Here's how the part is built. I have some questions about the finished solid (model axes, mm). Face numbers are marked on the shaded views. A direction names the side the tool comes from. Round coordinates to 2 decimals unless told otherwise and drop trailing zeros. Loops run counter-clockwise (first coordinate to the right, second up) from the corner with the lowest first, then second, coordinate; pieces in that order, holes last. Notation, with made-up numbers: (14, -33.5) - (66, -33.5) arc R22 ccw to (66, -9.5) - close; hole circle Ø2 at (78, 24.25). An arc over 180 degrees is marked (long way). Answer as a JSON object with one key per item and string values. Group by question number.
1) If I drill on line 1 along Z through (x, y) = (8.5, 1.05); line 2 along X through (y, z) = (21.5, -12.5) (3 decimals); line 3 along X through (y, z) = (17, -12) (3 decimals), over which ranges is the centre line in solid material (lowest first)? Write a range as [from, to].
2) Which directions (+Z, -Z, +X, -X, +Y, -Y) give clear straight access to the entire face, cutting with the end or side of a thin tool? Please do the marked faces 1, 2 and 3.
3) I want a section at A-A, the plane x = 0. Please give me the cut outline in (y, z).
4) I want a section at C-C, the plane z = 13. Please give me the cut outline in (x, y) (3 decimals).
5) I want a section at B-B, the plane y = 21.5. Please give me the cut outline in (x, z) (3 decimals).
6) Will these pins go through, and if not, where does the flat tip stop? P1, Ø5.5, axis at y = 17, z = 16, coming from the +X side (3 decimals); P2, Ø3.5, axis at x = -23.855, y = 20.644, coming from the -Z side; P3, Ø0.5, axis at x = 22.5, y = 1, coming from the +Z side; P4, Ø3.5, axis at x = 8.5, z = 3.08, coming from the +Y side.
7) I want a section at D-D, the plane x = 6.5. Please give me the cut outline in (y, z), then the cut area to 3 significant figures.
from build123d import *

# Parameters (mm, degrees)
SKETCH1_W               = 57.15
SKETCH1_H               = 34.72
BOSS_EXTRUDE1_DEPTH     = 1.524
SKETCH2_W               = 9.44
SKETCH2_H               = 4.95
CUT_EXTRUDE1_DEPTH      = 5
SKETCH3_R               = 2.1844
CUT_EXTRUDE2_DEPTH      = 5
SKETCH4_W               = 38.27
SKETCH4_H               = 1.524
SKETCH4_W_2             = 9.44
BOSS_EXTRUDE2_DEPTH     = 24.2
SKETCH5_R               = 1.59
CUT_EXTRUDE3_DEPTH      = 12.1
SKETCH6_R               = 1.09
CUT_EXTRUDE4_DEPTH      = 24.2
SKETCH7_R               = 4
CUT_EXTRUDE5_DEPTH      = 24.2
SKETCH8_R               = 1.09
CUT_EXTRUDE6_DEPTH      = 24.2
CIRPATTERN1_COUNT       = 4
MIRROR3_COPY_1_SKETCH_R = 1.09
MIRROR3_COPY_1_DEPTH    = 24.2
MIRROR3_COPY_2_SKETCH_R = 1.09
MIRROR3_COPY_2_DEPTH    = 24.2
SKETCH9_R               = 2.1844
CUT_EXTRUDE7_DEPTH      = 12.1
FILLET1_R               = 2
FILLET2_R               = 1


with BuildPart() as part:
    # Sketch1 → Boss-Extrude1 (new body)
    with BuildSketch(Plane(origin=(0, 0, 0), x_dir=(1, 0, 0), z_dir=(0, 1, 0))):
        Rectangle(SKETCH1_W, SKETCH1_H)
    extrude(amount=BOSS_EXTRUDE1_DEPTH)

    # Sketch2 → Cut-Extrude1 (cut, symmetric)
    with BuildSketch(Plane(origin=(0, 1.524, 0), x_dir=(1, 0, 0), z_dir=(0, 1, 0))):
        with Locations((23.855, -14.885)):
            Rectangle(SKETCH2_W, SKETCH2_H)
        Polygon((28.575, 17.36), (17.445, 17.36), (17.445, 8.41), (19.135, 8.41), (19.135, 13.36), (28.575, 13.36), align=None)
    cut_extrude1 = extrude(amount=CUT_EXTRUDE1_DEPTH, both=True, mode=Mode.SUBTRACT)

    # Mirror1: Cut-Extrude1 across plane
    add(cut_extrude1.mirror(Plane(origin=(0, 0, 0), x_dir=(0, 0, 1), z_dir=(1, 0, 0))), mode=Mode.SUBTRACT)

    # Sketch3 → Cut-Extrude2 (cut, symmetric)
    with BuildSketch(Plane(origin=(0, 1.524, 0), x_dir=(1, 0, 0), z_dir=(0, 1, 0))):
        with Locations(Location((23.855, -4.38, 0), (0, 0, 90))):
            Circle(SKETCH3_R)
        with Locations(Location((23.855, 5.42, 0), (0, 0, 90))):
            Circle(SKETCH3_R)
    cut_extrude2 = extrude(amount=CUT_EXTRUDE2_DEPTH, both=True, mode=Mode.SUBTRACT)

    # Mirror2: Cut-Extrude2 across plane
    add(cut_extrude2.mirror(Plane(origin=(0, 0, 0), x_dir=(0, 0, 1), z_dir=(1, 0, 0))), mode=Mode.SUBTRACT)

    # Sketch4 → Boss-Extrude2 (add)
    with BuildSketch(Plane(origin=(0, 1.524, 0), x_dir=(1, 0, 0), z_dir=(0, 1, 0))):
        with Locations((0, -16.598)):
            Rectangle(SKETCH4_W, SKETCH4_H)
        with Locations((-23.855, 12.598)):
            Rectangle(SKETCH4_W_2, SKETCH4_H)
        with Locations((23.855, 12.598)):
            Rectangle(SKETCH4_W_2, SKETCH4_H)
    extrude(amount=BOSS_EXTRUDE2_DEPTH)

    # Sketch5 → Cut-Extrude3 (cut, symmetric)
    with BuildSketch(Plane.XY.offset(17.36)):
        with Locations((-9.93, 15.794)):
            Circle(SKETCH5_R)
        with Locations((9.93, 15.794)):
            Circle(SKETCH5_R)
    extrude(amount=CUT_EXTRUDE3_DEPTH, both=True, mode=Mode.SUBTRACT)

    # Sketch6 → Cut-Extrude4 (cut)
    with BuildSketch(Plane(origin=(0, 1.524, 0), x_dir=(1, 0, 0), z_dir=(0, 1, 0))):
        with Locations(Location((0, 5.42, 0), (0, 0, 270))):
            Circle(SKETCH6_R)
    extrude(amount=-CUT_EXTRUDE4_DEPTH, mode=Mode.SUBTRACT)

    # Sketch7 → Cut-Extrude5 (cut)
    with BuildSketch(Plane(origin=(0, 1.524, 0), x_dir=(1, 0, 0), z_dir=(0, 1, 0))):
        with Locations(Location((-8.5, 5.42, 0), (0, 0, 270))):
            Circle(SKETCH7_R)
    cut_extrude5 = extrude(amount=-CUT_EXTRUDE5_DEPTH, mode=Mode.SUBTRACT)

    # Sketch8 → Cut-Extrude6 (cut)
    with BuildSketch(Plane(origin=(0, 1.524, 0), x_dir=(1, 0, 0), z_dir=(0, 1, 0))):
        with Locations(Location((-8.5, 13.92, 0), (0, 0, 270))):
            Circle(SKETCH8_R)
    cut_extrude6 = extrude(amount=-CUT_EXTRUDE6_DEPTH, mode=Mode.SUBTRACT)

    # CirPattern1: Cut-Extrude6 ×4 about axis, 1 skipped
    cirpattern1_axis = Axis((-8.5, 0, -5.42), (0, 1, 0))
    add([cut_extrude6.rotate(cirpattern1_axis, i * 360 / CIRPATTERN1_COUNT) for i in range(1, CIRPATTERN1_COUNT) if i not in (3,)], mode=Mode.SUBTRACT)

    # Mirror3: Cut-Extrude5, Cut-Extrude6 across plane
    add(cut_extrude5.mirror(Plane(origin=(0, 0, 0), x_dir=(0, 0, 1), z_dir=(1, 0, 0))), mode=Mode.SUBTRACT)
    add(cut_extrude6.mirror(Plane(origin=(0, 0, 0), x_dir=(0, 0, 1), z_dir=(1, 0, 0))), mode=Mode.SUBTRACT)

    # Mirror3 copy 1 sketch → Mirror3 copy 1 (cut)
    with BuildSketch(Plane(origin=(3.08, 1.524, -13.92), x_dir=(0, 0, -1), z_dir=(0, 1, 0))):
        with Locations((-8.5, -13.92)):
            Circle(MIRROR3_COPY_1_SKETCH_R)
    extrude(amount=-MIRROR3_COPY_1_DEPTH, mode=Mode.SUBTRACT)

    # Mirror3 copy 2 sketch → Mirror3 copy 2 (cut)
    with BuildSketch(Plane(origin=(17, 1.524, -10.84), x_dir=(1, 0, 0), z_dir=(0, 1, 0))):
        with Locations((-8.5, -13.92)):
            Circle(MIRROR3_COPY_2_SKETCH_R)
    extrude(amount=-MIRROR3_COPY_2_DEPTH, mode=Mode.SUBTRACT)

    # Sketch9 → Cut-Extrude7 (cut, symmetric)
    with BuildSketch(Plane.XY.offset(-11.836)):
        with Locations(Location((-23.855, 20.644, 0), (0, 0, 180))):
            Circle(SKETCH9_R)
        with Locations(Location((-23.855, 10.734, 0), (0, 0, 180))):
            Circle(SKETCH9_R)
        with Locations((23.855, 10.734)):
            Circle(SKETCH9_R)
        with Locations((23.855, 20.644)):
            Circle(SKETCH9_R)
    extrude(amount=CUT_EXTRUDE7_DEPTH, both=True, mode=Mode.SUBTRACT)

    # Fillet1
    fillet1_edges = [part.edges().sort_by_distance(p)[0] for p in [
        (28.575, 0.762, 12.41),
        (-28.575, 0.762, 12.41),
    ]]
    fillet(fillet1_edges, radius=FILLET1_R)

    # Fillet2
    fillet2_edges = [part.edges().sort_by_distance(p)[0] for p in [
        (0, 0, 17.36),
        (23.855, 0, -13.36),
        (-23.855, 0, -13.36),
        (0, 1.524, 15.836),
        (23.855, 1.524, -11.836),
        (-23.855, 1.524, -11.836),
    ]]
    fillet(fillet2_edges, radius=FILLET2_R)


solid = part.part
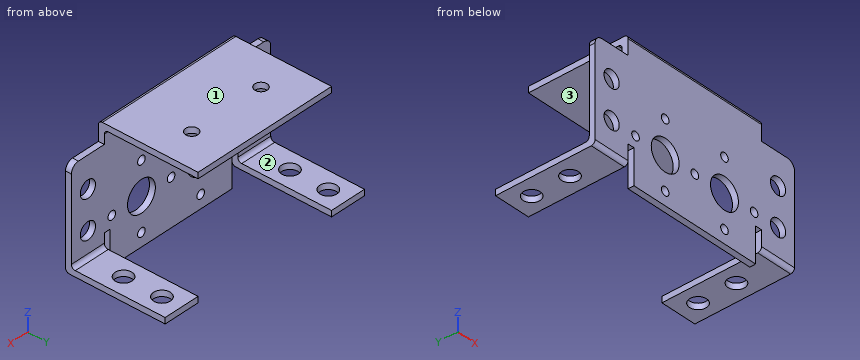
Outcome:
{
 "1": {"line 1": "[-17.36, -15.01], [-12.83, -9.42], [-1.42, 1.99], [4.17, 17.36]", "line 2": "[-28.575, -25.865], [-21.845, -19.135], [19.135, 21.845], [25.865, 28.575]", "line 3": "[-28.575, -19.135], [19.135, 28.575]"},
 "2": {"face 1": "+Z, +X, -X, +Y, -Y", "face 2": "+Z, +X, -X, +Y", "face 3": "-Z, +X, -X, +Y"},
 "3": {"outline": "(0, -17.36) - (1.52, -17.36) - (1.52, -6.51) - (0, -6.51) - close; (0, -4.33) - (1.52, -4.33) - (1.52, 14.84) arc R1 cw to (2.52, 15.84) - (25.72, 15.84) - (25.72, 17.36) - (1, 17.36) arc R1 ccw to (0, 16.36) - close"},
 "4": {"outline": "(-19.135, 0) - (19.135, 0) - (19.135, 1.524) - (-19.135, 1.524) - close"},
 "5": {"outline": "(-28.575, -13.36) - (-25.865, -13.36) - (-25.865, -11.836) - (-28.575, -11.836) - close; (-21.845, -13.36) - (-19.135, -13.36) - (-19.135, -11.836) - (-21.845, -11.836) - close; (-19.135, 15.836) - (19.135, 15.836) - (19.135, 17.36) - (-19.135, 17.36) - close; (19.135, -13.36) - (21.845, -13.36) - (21.845, -11.836) - (19.135, -11.836) - close; (25.865, -13.36) - (28.575, -13.36) - (28.575, -11.836) - (25.865, -11.836) - close"},
 "6": {"P1": "x = 19.135", "P2": "through", "P3": "z = 12.41", "P4": "y = 1.52"},
 "7": {"outline": "(0, -17.36) - (1.52, -17.36) - (1.52, -8.88) - (0, -8.88) - close; (0, -1.96) - (1.52, -1.96) - (1.52, 14.84) arc R1 cw to (2.52, 15.84) - (25.72, 15.84) - (25.72, 17.36) - (1, 17.36) arc R1 ccw to (0, 16.36) - close", "area": "79.2 mm^2"}
}
